from build123d import *

# Parameters (mm, degrees)
SKETCH_1_W          = 104
SKETCH_1_H          = 38
EXTRUDE_1_DEPTH     = 3
SKETCH_2_W          = 104
SKETCH_2_H          = 2
EXTRUDE_3_DEPTH     = 104
FILLET_1_R          = 3
CUT_EXTRUDE_1_DEPTH = 125.887949779


with BuildPart() as part:
    # 草图1 → 凸台-拉伸1 (new body)
    with BuildSketch(Plane(origin=(0, 0, 0), x_dir=(1, 0, 0), z_dir=(0, 1, 0))):
        Rectangle(SKETCH_1_W, SKETCH_1_H)
    extrude(amount=EXTRUDE_1_DEPTH)

    # 草图2 → 凸台-拉伸3 (add)
    with BuildSketch(Plane(origin=(0, 3, 0), x_dir=(1, 0, 0), z_dir=(0, 1, 0))):
        with Locations((0, 18)):
            Rectangle(SKETCH_2_W, SKETCH_2_H)
    extrude(amount=EXTRUDE_3_DEPTH)

    # 圆角1
    fillet_1_edges = [part.edges().sort_by_distance(p)[0] for p in [
        (0, 3, -17),
        (0, 0, -19),
    ]]
    fillet(fillet_1_edges, radius=FILLET_1_R)

    # 草图4 → 切除-拉伸1 (cut, through all)
    with BuildSketch(Plane(origin=(0, 0, -19), x_dir=(-1, 0, 0), z_dir=(0, 0, -1))):
        with BuildLine():
            Line((-5.452089617, 106.154609435), (4.543778851, 106.154609435))
            ThreePointArc((4.543778851, 106.154609435), (7.543778851, 103.154609435), (4.543778851, 100.154609435))
            Line((4.543778851, 100.154609435), (-5.452089617, 100.154609435))
            ThreePointArc((-5.452089617, 100.154609435), (-8.452089617, 103.154609435), (-5.452089617, 106.154609435))
        make_face()
    extrude(amount=-CUT_EXTRUDE_1_DEPTH, mode=Mode.SUBTRACT)


solid = part.part
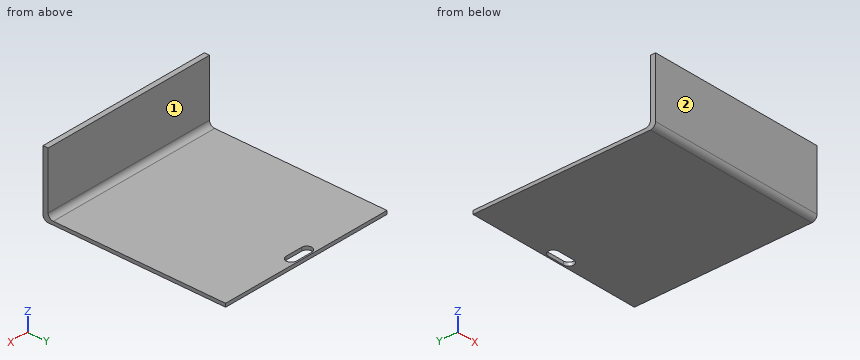
Verification items for the finished model (mm, model axes). Face numbers are marked on the shaded views. A direction names the side the tool comes from. Round coordinates to 2 decimals unless told otherwise and drop trailing zeros. Write each loop counter-clockwise with the first axis right and the second up, starting at its lowest first coordinate (ties: lowest second). Pieces come first, ordered by that corner, then holes.
(1) Section check B-B (y = 96). Enter the section's corners in (x, z), plus the area to 3 significant figures.
Returned:
outline: (-52, -19) - (52, -19) - (52, -17) - (-52, -17) - close
area: 208 mm2
(2) Material ranges on line 1 (Y direction, x = 3, z = -2.5); line 2 (Z direction, x = 24.5, y = 66.5), recorded low to high.
Returned:
line 1: y = 0 to 3
line 2: z = -19 to -17
(3) Section check C-C (z = -2.5). Enter the section's corners in (x, y).
Returned:
outline: (-52, 0) - (52, 0) - (52, 3) - (-52, 3) - close
(4) Access from +Z, -Z, +X, -X, +Y, -Y to the whole of each face (thin tool, end or side, straight path). Record for the marked faces 1 and 2.
Returned:
face 1: +Z, +X, -X, +Y
face 2: +Z, -Z, +X, -X, -Y
(5) Depth check by flat-ended pin: pin 1 Ø6 at (x, z) = (-26, 12) entering from +Y; pin 2 Ø8 at (x, y) = (-38, 38) entering from +Z; pin 3 Ø1 at (x, z) = (2, -18.5) entering from -Y. Enter the tip coordinate at first touch or a pass-through.
Returned:
pin 1: stops at y = 3
pin 2: stops at z = -17
pin 3: stops at y = 0.76
(6) Section check A-A (x = 12). Enter the section's corners in (y, z).
Returned:
outline: (0, -16) arc R3 ccw to (3, -19) - (107, -19) - (107, -17) - (6, -17) arc R3 cw to (3, -14) - (3, 19) - (0, 19) - close
